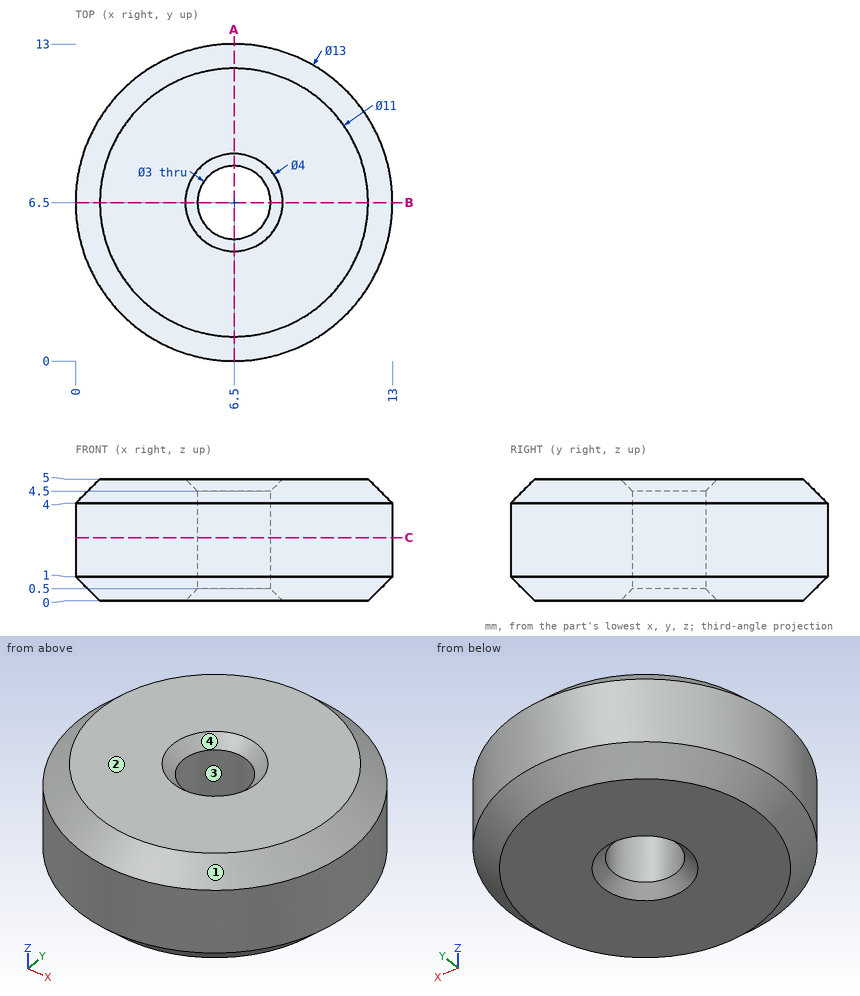
Part print with two shaded views. Sizes in mm from the minimum x, y, z corner. Round coordinates to 2 decimals unless told otherwise and drop trailing zeros. Order: outer loops, then holes, each group sorted by start corner. A loop starts at its lowest first (then second) coordinate and runs counter-clockwise, first axis right, second up. Notation, with made-up numbers: (9, 68) -> (24, 68) arc R19 cw to (24, 84) -> close; hole circle Ø2 at (-26.5, 74.25). An arc over 180 degrees is marked (long way). Write each question's results on one line, items separated by ' | '.
1. Cut at A-A (x = 6.5). Give the cut face in (y, z).
Findings below:
outline: (0, 1) -> (1, 0) -> (4.5, 0) -> (5, 0.5) -> (5, 4.5) -> (4.5, 5) -> (1, 5) -> (0, 4) -> close; (8, 0.5) -> (8.5, 0) -> (12, 0) -> (13, 1) -> (13, 4) -> (12, 5) -> (8.5, 5) -> (8, 4.5) -> close
2. Pull direction X, two halves, no side cores. Call the marked faces 1, 2, 3 and 4: pulls with the +X half, pulls with the -X half, needs draft (parallel to the pull), parting line crosses it, or undercut.
Findings below:
face 1: parting line crosses it | face 2: needs draft | face 3: undercut | face 4: undercut
3. Flat gauge pin, fed straight in: P1, Ø2.5, axis at x = 6.5, y = 6.5, coming from the +Z side. Where does the tip first touch, or does it go through?
Findings below:
P1: passes through
4. Wall check: line 1 along Y through (x, z) = (6.5, 2.55); line 2 along X through (y, z) = (6.25, 3.2); line 3 along Z through (x, y) = (5.75, 5). Give the ranges that are in metal, low to high. Write a range as [from, to].
Findings below:
line 1: y = [0, 5], [8, 13] | line 2: x = [0, 5.02], [7.98, 13] | line 3: z = [0.32, 4.68]
5. Cut at C-C (z = 2.6). Give the cut face in (x, y).
Findings below:
outline: circle Ø13 at (6.5, 6.5); hole circle Ø3 at (6.5, 6.5)
